Geometry check sheet. Reference: drawing and pictorial views, mm from the part's lowest x, y, z. Round coordinates to 2 decimals unless told otherwise and drop trailing zeros. Order: outer loops, then holes, each group sorted by start corner. A loop starts at its lowest first (then second) coordinate and runs counter-clockwise, first axis right, second up.
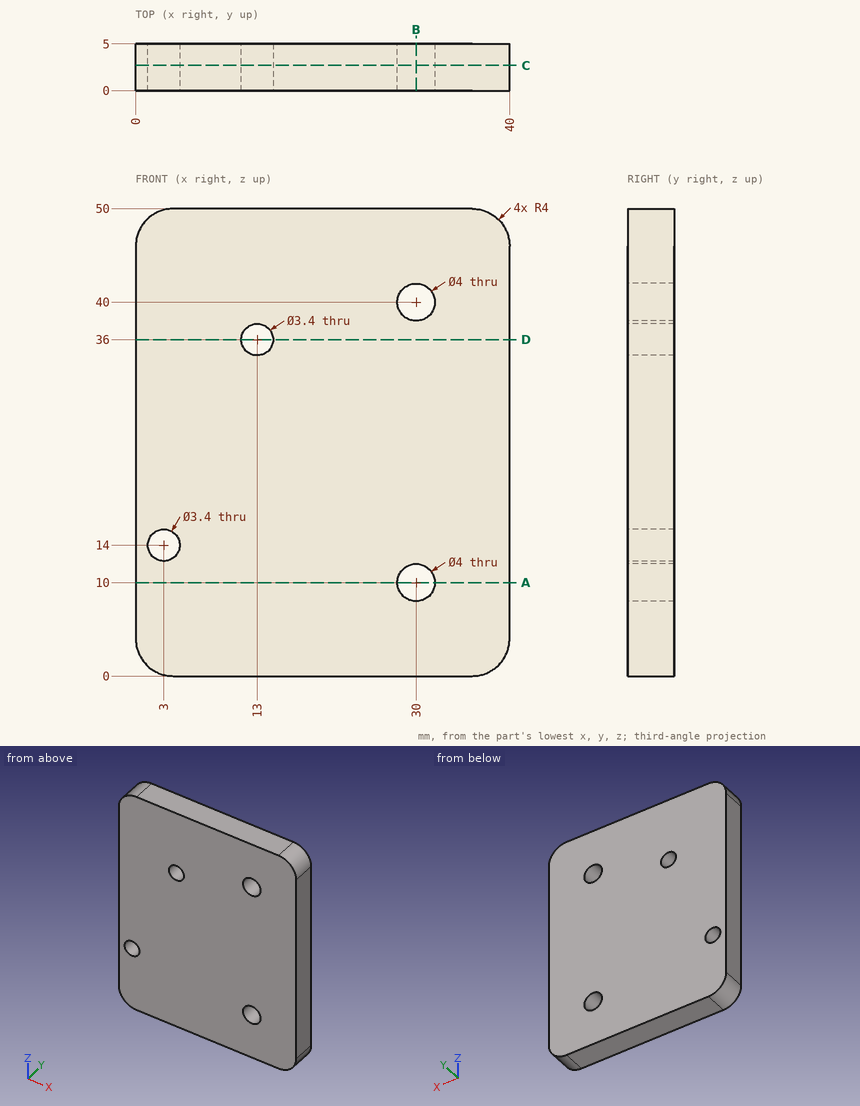
1) Sectioned sample at A-A on z = 10. Record the cut outline in (x, y).
2) Scan lines: probe 1 along Z at (x, y) = (30, 1.35); probe 2 along Z at (x, y) = (29, 4.2); probe 3 along Z at (x, y) = (13, 3.75). Record each from-to range of solid material in increasing order.
3) Sectioned sample at D-D on z = 36. Record the cut outline in (x, y), then the cut area to 3 significant figures.
4) Sectioned sample at C-C on y = 2.7. Record the cut outline in (x, z).
5) Sectioned sample at B-B on x = 30. Record the cut outline in (y, z).
6) Go/stop test with a flat-tipped pin: pin 1 Ø3.5 at (x, z) = (30, 10) entering from +Y. Record where the tip stops, or that it passes through.
Returned:
1. outline: (0, 0) - (28, 0) - (28, 5) - (0, 5) - close; (32, 0) - (40, 0) - (40, 5) - (32, 5) - close
2. probe 1: z = 0 to 8, 12 to 38, 42 to 50
2. probe 2: z = 0 to 8.27, 11.73 to 38.27, 41.73 to 50
2. probe 3: z = 0 to 34.3, 37.7 to 50
3. outline: (0, 0) - (11.3, 0) - (11.3, 5) - (0, 5) - close; (14.7, 0) - (40, 0) - (40, 5) - (14.7, 5) - close
3. area: 183 mm2
4. outline: (0, 4) arc R4 ccw to (4, 0) - (36, 0) arc R4 ccw to (40, 4) - (40, 46) arc R4 ccw to (36, 50) - (4, 50) arc R4 ccw to (0, 46) - close; hole circle Ø3.4 at (3, 14); hole circle Ø3.4 at (13, 36); hole circle Ø4 at (30, 10); hole circle Ø4 at (30, 40)
5. outline: (0, 0) - (5, 0) - (5, 8) - (0, 8) - close; (0, 12) - (5, 12) - (5, 38) - (0, 38) - close; (0, 42) - (5, 42) - (5, 50) - (0, 50) - close
6. pin 1: passes through
